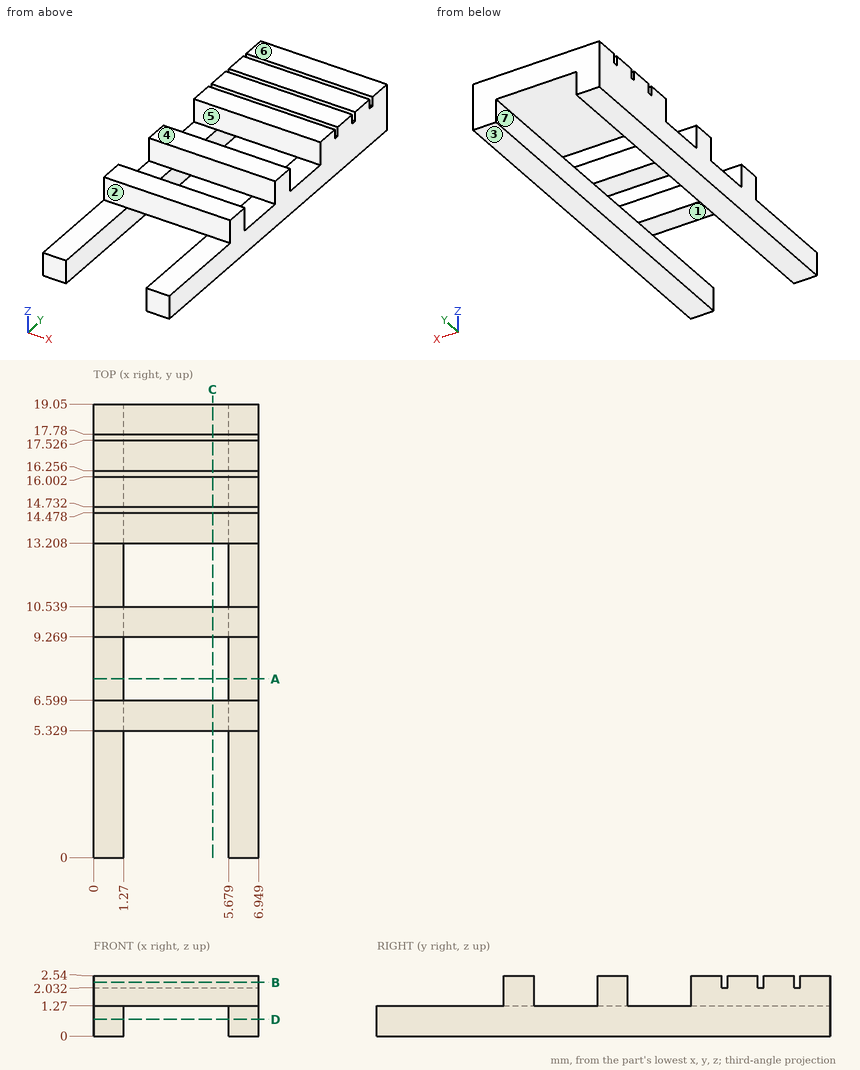
Print and shaded views of the part. All mm, measured from the part's lowest x, y and z. A direction names the side the tool comes from. Coordinates: 2 decimals unless noted, no trailing zeros. Write each loop counter-clockwise with the first axis right and the second up, starting at its lowest first coordinate (ties: lowest second). Pieces come first, ordered by that corner, then holes.
(1) Drill centre lines: probe 1 along Y at (x, z) = (3.5, 1.35); probe 2 along Y at (x, z) = (3.75, 2.3); probe 3 along X at (y, z) = (13.75, 1.05). Where is each one in solid material? Low to high.
(2) Flat gauge pins, fed straight in: pin 1 (0.6 mm diameter, centred on x = 6, y = 12.5, fed in from +Z); pin 2 (0.6 mm diameter, centred on x = 4.5, z = 2.5, fed in from -Y); pin 3 (1.4 mm diameter, centred on x = 4.5, y = 10, fed in from -Z). Where does each tip first touch, or does it go through?
(3) Cut at B-B, the plane z = 2.25. List the corners of the cut face in (x, y).
(4) Cut at C-C, the plane x = 5. List the corners of the cut face in (y, z).
(5) Cut at A-A, the plane y = 7.5. List the corners of the cut face in (x, z).
(6) Two-plate mould, pull along X, no slides. Class the marked faces 6 and 7: +X half, -X half, draft (parallel to the pull), parting line (faces both ways), or undercut.
(7) 3-axis set-ups, long thin cutter, end or side, ignore diameter. For the marked faces 1, 2, 3, 4 and 5: which of +Z, -Z, +X, -X, +Y, -Y reach the whole face in a straight line?
(8) Cut at D-D, the plane z = 0.7. List the corners of the cut face in (x, y).
Geometry says:
1. probe 1: y = 5.33 to 6.6, 9.27 to 10.54, 13.21 to 19.05
1. probe 2: y = 5.33 to 6.6, 9.27 to 10.54, 13.21 to 14.48, 14.73 to 16, 16.26 to 17.53, 17.78 to 19.05
1. probe 3: x = 0 to 1.27, 5.68 to 6.95
2. pin 1: stops at z = 1.27
2. pin 2: stops at y = 5.33
2. pin 3: stops at z = 1.27
3. outline: (0, 5.33) - (6.95, 5.33) - (6.95, 6.6) - (0, 6.6) - close; (0, 9.27) - (6.95, 9.27) - (6.95, 10.54) - (0, 10.54) - close; (0, 13.21) - (6.95, 13.21) - (6.95, 14.48) - (0, 14.48) - close; (0, 14.73) - (6.95, 14.73) - (6.95, 16) - (0, 16) - close; (0, 16.26) - (6.95, 16.26) - (6.95, 17.53) - (0, 17.53) - close; (0, 17.78) - (6.95, 17.78) - (6.95, 19.05) - (0, 19.05) - close
4. outline: (5.33, 1.27) - (6.6, 1.27) - (6.6, 2.54) - (5.33, 2.54) - close; (9.27, 1.27) - (10.54, 1.27) - (10.54, 2.54) - (9.27, 2.54) - close; (13.21, 1.27) - (19.05, 1.27) - (19.05, 2.54) - (17.78, 2.54) - (17.78, 2.03) - (17.53, 2.03) - (17.53, 2.54) - (16.26, 2.54) - (16.26, 2.03) - (16, 2.03) - (16, 2.54) - (14.73, 2.54) - (14.73, 2.03) - (14.48, 2.03) - (14.48, 2.54) - (13.21, 2.54) - close
5. outline: (0, 0) - (1.27, 0) - (1.27, 1.27) - (0, 1.27) - close; (5.68, 0) - (6.95, 0) - (6.95, 1.27) - (5.68, 1.27) - close
6. face 6: draft
6. face 7: undercut
7. face 1: -Z, +Y, -Y
7. face 2: +Z, +X, -X, -Y
7. face 3: -Z, +X, -X, +Y, -Y
7. face 4: +Z, +X, -X, +Y, -Y
7. face 5: +Z, +X, -X
8. outline: (0, 0) - (1.27, 0) - (1.27, 19.05) - (0, 19.05) - close; (5.68, 0) - (6.95, 0) - (6.95, 19.05) - (5.68, 19.05) - close
